Build history of the part. All positions in model axes, mm. A direction names the side the tool comes from. Coordinates: 2 decimals unless noted, no trailing zeros. Loops run counter-clockwise (first coordinate to the right, second up) from the corner with the lowest first, then second, coordinate; pieces in that order, holes last. Notation, with made-up numbers: M 46,76 L 88,76 A28 ccw 88,102 Z; hole C 74.5,78 d9. An arc over 180 degrees is marked long. Write each question's results on one line, items separated by ' | '. Start each with the question number.
from build123d import *

# Parameters (mm, degrees)
EXTRUDE_1_DEPTH     = 2
SKETCH_3_R          = 2.5
EXTRUDE_2_DEPTH     = 0.8
EXTRUDE_START       = 1.5
SKETCH_4_R          = 3
EXTRUDE_3_DEPTH     = 1.5
SKETCH_5_R          = 2
CUT_EXTRUDE_1_DEPTH = 2.8
CUT_EXTRUDE_START   = -0.8
SKETCH_6_R          = 2
CUT_EXTRUDE_2_DEPTH = 0.8
SKETCH_7_R          = 1
CUT_EXTRUDE_3_DEPTH = 17.170961629
SKETCH_8_R          = 0.775
CUT_EXTRUDE_4_DEPTH = 17.170961629


with BuildPart() as part:
    # Эскиз2 → Бобышка-Вытянуть1 (new body)
    with BuildSketch(Plane(origin=(0, 0, 0), x_dir=(1, 0, 0), z_dir=(0, 1, 0))):
        with BuildLine():
            ThreePointArc((0.4420191, 2.967257844), (2.272229885, 1.958818866), (3, 0))
            Line((3, 0), (11.5, 0))
            ThreePointArc((11.5, 0), (12.085786438, 1.414213562), (13.5, 2))
            Line((13.5, 2), (0.4420191, 2.967257844))
        make_face()
        with BuildLine():
            ThreePointArc((0, 3), (-2.121320344, 2.121320344), (-3, 0))
            Line((-3, 0), (3, 0))
            ThreePointArc((3, 0), (2.272229885, 1.958818866), (0.4420191, 2.967257844))
            Line((0.4420191, 2.967257844), (0, 3))
        make_face()
        with BuildLine():
            Line((3, 0), (-3, 0))
            ThreePointArc((-3, 0), (-2.121320344, -2.121320344), (0, -3))
            Line((0, -3), (0.4420191, -2.967257844))
            ThreePointArc((0.4420191, -2.967257844), (2.272229885, -1.958818866), (3, 0))
        make_face()
        with BuildLine():
            Line((11.5, 0), (3, 0))
            ThreePointArc((3, 0), (2.272229885, -1.958818866), (0.4420191, -2.967257844))
            Line((0.4420191, -2.967257844), (13.5, -2))
            ThreePointArc((13.5, -2), (12.085786438, -1.414213562), (11.5, 0))
        make_face()
        with BuildLine():
            ThreePointArc((13.5, 2), (12.085786438, 1.414213562), (11.5, 0))
            Line((11.5, 0), (15.5, 0))
            ThreePointArc((15.5, 0), (14.914213562, 1.414213562), (13.5, 2))
        make_face()
        with BuildLine():
            Line((15.5, 0), (11.5, 0))
            ThreePointArc((11.5, 0), (12.085786438, -1.414213562), (13.5, -2))
            ThreePointArc((13.5, -2), (14.914213562, -1.414213562), (15.5, 0))
        make_face()
    extrude(amount=EXTRUDE_1_DEPTH)

    # Эскиз3 → Бобышка-Вытянуть2 (add)
    with BuildSketch(Plane(origin=(0, 2, 0), x_dir=(1, 0, 0), z_dir=(0, 1, 0))):
        with Locations(Location((0, 0, 0), (0, 0, 270))):
            Circle(SKETCH_3_R)
    extrude(amount=EXTRUDE_2_DEPTH)

    # Эскиз4 → Бобышка-Вытянуть3 (add)
    with BuildSketch(Plane.XZ.offset(EXTRUDE_START)):
        with Locations(Location((0, 0, 0), (0, 0, 270))):
            Circle(SKETCH_4_R)
    extrude(amount=-EXTRUDE_3_DEPTH)

    # Эскиз5 → Вырез-Вытянуть1 (cut)
    with BuildSketch(Plane(origin=(0, -1.5, 0), x_dir=(-1, 0, 0), z_dir=(0, -1, 0))):
        with Locations(Location((0, 0, 0), (0, 0, 90))):
            Circle(SKETCH_5_R)
    extrude(amount=-CUT_EXTRUDE_1_DEPTH, mode=Mode.SUBTRACT)

    # Эскиз6 → Вырез-Вытянуть2 (cut)
    with BuildSketch(Plane(origin=(0, 2.8, 0), x_dir=(1, 0, 0), z_dir=(0, 1, 0)).offset(CUT_EXTRUDE_START)):
        with Locations(Location((0, 0, 0), (0, 0, 90))):
            Circle(SKETCH_6_R)
    extrude(amount=CUT_EXTRUDE_2_DEPTH, mode=Mode.SUBTRACT)

    # Эскиз7 → Вырез-Вытянуть3 (cut, through all)
    with BuildSketch(Plane(origin=(0, 2, 0), x_dir=(1, 0, 0), z_dir=(0, 1, 0))):
        with Locations(Location((0, 0, 0), (0, 0, 270))):
            Circle(SKETCH_7_R)
    extrude(amount=-CUT_EXTRUDE_3_DEPTH, mode=Mode.SUBTRACT)

    # Эскиз8 → Вырез-Вытянуть4 (cut, through all)
    with BuildSketch(Plane(origin=(0, 2, 0), x_dir=(1, 0, 0), z_dir=(0, 1, 0))):
        with Locations(Location((9.5, 0, 0), (0, 0, 270))):
            Circle(SKETCH_8_R)
    extrude(amount=-CUT_EXTRUDE_4_DEPTH, mode=Mode.SUBTRACT)


solid = part.part
1. Band-saw the part on C-C, the plane z = -0.4. List the corners of the cut face in (x, y).
2. Mould opens along Z. For faces 1 (the cylindrical face through (1.952, 2.394, 0.434)), 2 (the cylindrical face through (-2.44, 2.39, -0.54)), 3 (the cylindrical face through (-0.976, 1.655, -0.217)), 4 (the flat face through (2, 2.8, -1)) say: +Z half, -Z half, draft (parallel to the pull), parting line (faces both ways), or undercut.
3. Band-saw the part on A-A, the plane x = 9.5. List the corners of the cut face in (y, z) (3 decimals), plus the area to 3 significant figures.
4. Band-saw the part on B-B, the plane y = 1. List the corners of the cut face in (x, z) (3 decimals), plus the area to 3 significant figures.
5. Which spindle directions (+Z, -Z, +X, -X, +Y, -Y) get a long thin tool onto all of the face, cutting with end or side? Do faces 5 (the flat face through (1, 2, -1)), 6 (the cylindrical face through (-2, 0, 0)), 7 (the flat face through (-1, -1.5, -2)). Say none if no direction does.
6. Pin check, flat tips, straight feed: pin 1 (2 mm diameter, centred on x = 4, z = 1, fed in from +Y); pin 2 (1.2 mm diameter, centred on x = 9.5, z = 0, fed in from +Y); pin 3 (3.5 mm diameter, centred on x = 0, z = 0, fed in from -Y). Stop position of each tip, or through.
7. Band-saw the part on D-D, the plane y = 2.4. List the corners of the cut face in (x, z).
8. Wall check: line 1 along X through (y, z) = (0.9, 0) (3 decimals); line 2 along X through (y, z) = (1.85, 0) (3 decimals); line 3 along X through (y, z) = (2.55, 0). Give the ranges that are in metal, low to high.
Checked values:
1) outline: M -2.97,-1.5 L -1.96,-1.5 L -1.96,1.3 L -0.92,1.3 L -0.92,2 L -1.96,2 L -1.96,2.8 L -2.47,2.8 L -2.47,2 L -2.97,2 Z; M 0.92,1.3 L 1.96,1.3 L 1.96,-1.5 L 2.97,-1.5 L 2.97,0 L 8.84,0 L 8.84,2 L 2.47,2 L 2.47,2.8 L 1.96,2.8 L 1.96,2 L 0.92,2 Z; M 10.16,0 L 15.46,0 L 15.46,2 L 10.16,2 Z
2) face 1: undercut | face 2: parting line | face 3: undercut | face 4: draft
3) outline: M 0,-2.296 L 2,-2.296 L 2,-0.775 L 0,-0.775 Z; M 0,0.775 L 2,0.775 L 2,2.296 L 0,2.296 Z | area: 6.09 mm²
4) outline: M 0,-3 L 13.5,-2 A2 ccw 13.5,2 L 0,3 A3 ccw Z; hole C 0,0 d4; hole C 9.5,0 d1.55 | area: 73.5 mm²
5) face 5: +Y | face 6: -Y | face 7: +Z, -Z, +X, -X, -Y
6) pin 1: y = 2 | pin 2: through | pin 3: y = 1.3
7) outline: C 0,0 d5; hole C 0,0 d4
8) line 1: -3 to -2, 2 to 8.725, 10.275 to 15.5 | line 2: -3 to -1, 1 to 8.725, 10.275 to 15.5 | line 3: -2.5 to -2, 2 to 2.5
